Check sheet for the modelled part. Datum: model origin and axes. Units: mm. A direction names the side the tool comes from. Round coordinates to 2 decimals unless told otherwise and drop trailing zeros. Write each loop counter-clockwise with the first axis right and the second up, starting at its lowest first coordinate (ties: lowest second). Pieces come first, ordered by that corner, then holes. Notation, with made-up numbers: (-21, 38) - (8, 38) arc R14 cw to (8, 65) - close; hole circle Ø3 at (47, 55.25). An arc over 180 degrees is marked (long way). Answer as a JSON object with one key per item and string values. Group by question number.
Item 1: Sectioned sample at C-C on z = -17. Record the boundary of the cut face in (x, y).
Item 2: Sectioned sample at B-B on y = 1.5. Record the boundary of the cut face in (x, z).
Item 3: Thickness scan on line 1 (X direction, y = 7.25, z = -29); line 2 (X direction, y = 11.5, z = -30); line 3 (Z direction, x = 4.75, y = 4.5). Record the ranges inside material, lowest first.
Item 4: Gauge pin test, flat ends, axial feed: P1, Ø6, axis at x = 24, z = -29.5, coming from the +Y side; P2, Ø1.1, axis at x = 2, z = -5.5, coming from the +Y side; P3, Ø12, axis at x = 16, z = -13, coming from the -Y side; P4, Ø1, axis at x = 7, y = 17, coming from the -Z side. Record the tip position at first contact, or that the pin passes through.
Item 5: Sectioned sample at D-D on z = -28. Record the boundary of the cut face in (x, y), plus the area to 3 significant figures.
Item 6: Set-up check for faces 4 (the cylindrical face through (29.699, 17.215, -5.603)), 5 (the flat face through (24, 16, -25.25)), 6 (the flat face through (2, 17.5, -6)), 7 (the cylindrical face through (0.285, 11.56, -1.801)): record each of +Z, -Z, +X, -X, +Y, -Y from which the full face is reachable in a straight line by a thin tool's end or side.
Item 7: Sectioned sample at A-A on x = 24. Count the separate pieces of the cut face and the enclosed holes in it, plus the area to 3 significant figures.
Item 8: Release check for a two-part mould opening along Z. For faces 1 (the flat face through (20.67, 15.98, -3.27)), 2 (the flat face through (14.8, 19.73, -23.59)), 3 (the cylindrical face through (0.285, 21.699, -17.053)) record: pulls with the +Z half, pulls with the -Z half, needs draft (parallel to the pull), parting line crosses it, or undercut.
```python
from build123d import *

# Parameters (mm, degrees)
SKETCH1_W               = 30
SKETCH1_H               = 34
BOSS_EXTRUDE1_DEPTH     = 22
SKETCH2_R               = 2.05
CUT_EXTRUDE1_DEPTH      = 22
SKETCH3_R               = 7.55
CUT_EXTRUDE2_DEPTH      = 51.398412673
CUT_EXTRUDE3_DEPTH      = 3
CUT_EXTRUDE3_DEPTH_BACK = 3
FILLET1_R               = 1


with BuildPart() as part:
    # Sketch1 → Boss-Extrude1 (new body)
    with BuildSketch(Plane(origin=(0, 0, 0), x_dir=(1, 0, 0), z_dir=(0, 1, 0))):
        with Locations((15, 17)):
            Rectangle(SKETCH1_W, SKETCH1_H)
    extrude(amount=BOSS_EXTRUDE1_DEPTH)

    # Sketch2 → Cut-Extrude1 (cut)
    with BuildSketch(Plane(origin=(0, 22, 0), x_dir=(1, 0, 0), z_dir=(0, 1, 0))):
        with Locations(Location((6, 29, 0), (0, 0, 270))):
            Circle(SKETCH2_R)
        with Locations(Location((24, 29, 0), (0, 0, 270))):
            Circle(SKETCH2_R)
        with Locations(Location((24, 5, 0), (0, 0, 270))):
            Circle(SKETCH2_R)
        with Locations(Location((6, 5, 0), (0, 0, 270))):
            Circle(SKETCH2_R)
    extrude(amount=-CUT_EXTRUDE1_DEPTH, mode=Mode.SUBTRACT)

    # Sketch3 → Cut-Extrude2 (cut, through all)
    with BuildSketch(Plane.ZY):
        with BuildLine():
            Line((-34, 22), (-34, 5.5))
            Line((-34, 5.5), (-32.5, 7.804886114))
            Line((-32.5, 7.804886114), (-32.5, 15.5))
            ThreePointArc((-32.5, 15.5), (-31.914213562, 16.914213562), (-30.5, 17.5))
            Line((-30.5, 17.5), (-26.35296805, 17.5))
            ThreePointArc((-26.35296805, 17.5), (-25.492668875, 17.694484747), (-24.799684767, 18.240114671))
            Line((-24.799684767, 18.240114671), (-22.350315233, 21.259885329))
            ThreePointArc((-22.350315233, 21.259885329), (-21.657331125, 21.805515253), (-20.79703195, 22))
            Line((-20.79703195, 22), (-34, 22))
        make_face()
        with BuildLine():
            Line((0, 22), (-13.20296805, 22))
            ThreePointArc((-13.20296805, 22), (-12.342668875, 21.805515253), (-11.649684767, 21.259885329))
            Line((-11.649684767, 21.259885329), (-9.200315233, 18.240114671))
            ThreePointArc((-9.200315233, 18.240114671), (-8.507331125, 17.694484747), (-7.64703195, 17.5))
            Line((-7.64703195, 17.5), (-3.5, 17.5))
            ThreePointArc((-3.5, 17.5), (-2.085786438, 16.914213562), (-1.5, 15.5))
            Line((-1.5, 15.5), (-1.5, 7.804886114))
            Line((-1.5, 7.804886114), (0, 5.5))
            Line((0, 5.5), (0, 22))
        make_face()
        with Locations((-17, 11)):
            Circle(SKETCH3_R)
        Polygon((-22, 1), (-22.811111111, 0), (-11.188888889, 0), (-12, 1), align=None)
    extrude(amount=-CUT_EXTRUDE2_DEPTH, mode=Mode.SUBTRACT)

    # Sketch4 → Cut-Extrude3 (cut, two sides: drawn at the far end of the back side and taken through both)
    with BuildSketch(Plane(origin=(0, 17.5, 0), x_dir=(1, 0, 0), z_dir=(0, 1, 0)).offset(-CUT_EXTRUDE3_DEPTH_BACK)):
        Polygon((8.165063509, 32.75), (3.834936491, 32.75), (1.669872981, 29), (3.834936491, 25.25), (8.165063509, 25.25), (10.330127019, 29), align=None)
        Polygon((26.165063509, 32.75), (21.834936491, 32.75), (19.669872981, 29), (21.834936491, 25.25), (26.165063509, 25.25), (28.330127019, 29), align=None)
        Polygon((21.834936491, 1.25), (26.165063509, 1.25), (28.330127019, 5), (26.165063509, 8.75), (21.834936491, 8.75), (19.669872981, 5), align=None)
        Polygon((8.165063509, 1.25), (10.330127019, 5), (8.165063509, 8.75), (3.834936491, 8.75), (1.669872981, 5), (3.834936491, 1.25), align=None)
    extrude(amount=CUT_EXTRUDE3_DEPTH + CUT_EXTRUDE3_DEPTH_BACK, mode=Mode.SUBTRACT)

    # Fillet1
    fillet1_edges = [part.edges().sort_by_distance(p)[0] for p in [
        (0, 22, -17),
        (30, 22, -17),
        (0, 2.75, -34),
        (30, 2.75, -34),
        (30, 2.75, 0),
        (0, 2.75, 0),
        (0, 16.914213562, -2.085786438),
        (30, 17.5, -5.573515975),
        (0, 21.805515253, -12.342668875),
        (0, 6.652443057, -0.75),
        (0, 11.652443057, -1.5),
        (0, 17.694484747, -8.507331125),
        (30, 19.75, -10.425),
        (30, 21.805515253, -12.342668875),
        (30, 6.652443057, -0.75),
        (30, 11.652443057, -1.5),
        (30, 16.914213562, -2.085786438),
        (30, 17.694484747, -8.507331125),
        (0, 19.75, -10.425),
        (0, 17.5, -5.573515975),
        (30, 11, -24.55),
        (0, 11, -24.55),
        (30, 17.5, -28.426484025),
        (30, 16.914213562, -31.914213562),
        (0, 21.805515253, -21.657331125),
        (30, 19.75, -23.575),
        (30, 17.694484747, -25.492668875),
        (30, 11.652443057, -32.5),
        (30, 6.652443057, -33.25),
        (30, 21.805515253, -21.657331125),
        (0, 6.652443057, -33.25),
        (0, 11.652443057, -32.5),
        (0, 16.914213562, -31.914213562),
        (0, 17.5, -28.426484025),
        (0, 17.694484747, -25.492668875),
        (0, 19.75, -23.575),
    ]]
    fillet(fillet1_edges, radius=FILLET1_R)


solid = part.part
```
Completed:
{
 "1": {"outline": "(0, 1) - (30, 1) - (30, 2.45) arc R1 ccw to (29, 3.45) - (1, 3.45) arc R1 ccw to (0, 2.45) - close; (0, 19.55) arc R1 ccw to (1, 18.55) - (29, 18.55) arc R1 ccw to (30, 19.55) - (30, 21) arc R1 ccw to (29, 22) - (1, 22) arc R1 ccw to (0, 21) - close"},
 "2": {"outline": "(0, -33) arc R1 ccw to (1, -34) - (29, -34) arc R1 ccw to (30, -33) - (30, -1) arc R1 ccw to (29, 0) - (1, 0) arc R1 ccw to (0, -1) - close; hole circle Ø4.1 at (6, -29); hole circle Ø4.1 at (6, -5); hole circle Ø4.1 at (24, -29); hole circle Ø4.1 at (24, -5)"},
 "3": {"line 1": "0 to 3.95, 8.05 to 21.95, 26.05 to 30", "line 2": "0 to 4.21, 7.79 to 22.21, 25.79 to 30", "line 3": "-34 to -30.62, -27.38 to -20.84, -13.16 to -6.62, -3.38 to 0"},
 "4": {"P1": "y = 14.5", "P2": "y = 17.5", "P3": "y = 0", "P4": "z = -25.25"},
 "5": {"outline": "(0, 0) - (4.21, 0) - (4.21, 14.5) - (2.25, 14.5) - (2.25, 17.5) - (1, 17.5) arc R1 ccw to (0, 16.5) - close; (7.79, 0) - (22.21, 0) - (22.21, 14.5) - (20.25, 14.5) - (20.25, 17.5) - (9.75, 17.5) - (9.75, 14.5) - (7.79, 14.5) - close; (25.79, 0) - (30, 0) - (30, 16.5) arc R1 ccw to (29, 17.5) - (27.75, 17.5) - (27.75, 14.5) - (25.79, 14.5) - close", "area": "376 mm²"},
 "6": {"face 4": "+Z, +X, +Y", "face 5": "-Z, +Y", "face 6": "+Z, +X, -X, +Y", "face 7": "+Z, -X, +Y"},
 "7": {"separate pieces": "3", "enclosed holes": "1", "area": "269 mm²"},
 "8": {"face 1": "undercut", "face 2": "pulls with the -Z half", "face 3": "needs draft"}
}
